Read the model definition and answer for the solid it produces. Units are mm, in the model's axes. A direction names the side the tool comes from. Give positions to 0.01 mm unless a question says otherwise; leave off trailing zeros. Order: outer loops, then holes, each group sorted by start corner. A loop starts at its lowest first (then second) coordinate and runs counter-clockwise, first axis right, second up.
Item 1: The mould has two halves that part along Y. Classify faces 3 (the face through (-35, -635, 1)), 4 (the face through (-26, 381, 12.7)), 5 (the face through (-28, -9, 6.35)), 6 (the face through (-35, 635, 1)): +Y half, -Y half, draft (parallel to the pull), parting line (faces both ways), or undercut.
Item 2: Given pin 1 Ø12.5 at (y, z) = (125, -14) entering from +X; pin 2 Ø1.5 at (x, y) = (-39.5, 37.5) entering from -Z; pin 3 Ø5 at (x, y) = (-39.5, 440.5) entering from +Z, each flat-ended and moving along its own axis, determine where each tip first touches the part or whether it passes through.
Item 3: A cutting plane is placed at B-B (z = -9). Write down the section's boundary in (x, y), plus the area to 3 significant figures.
Item 4: A cutting plane is placed at A-A (y = -316.5). Write down the section's boundary in (x, z), plus the area to 3 significant figures.
Item 5: Which of the six approach directions +Z, -Z, +X, -X, +Y, -Y give full straight-line access (tool end or side, diameter ignored) to faces 1 (the face through (-50.8, -9, -13)), 2 (the face through (-26, -381, 12.7))?
Item 6: Find the intervals of material crossed by line 1 along X through (y, z) = (466.5, -13); line 2 along Z through (x, y) = (-6, 179.5); line 3 along Y through (x, z) = (-35, 11), in increasing order.
from build123d import *

# Parameters (mm, degrees)
F1_DEPTH = 635
F2_R     = 12.7
F3_DEPTH = 12.7


# Not quite as in the source:
# - a fillet or chamfer that OpenCascade refuses, or shapes differently, is made with other operations: its cross-section is extruded or revolved along the edge and cut away or added


with BuildPart() as f1:
    # F0 (on Front) → F1 (new body, symmetric)
    with BuildSketch(Plane.XZ):
        Polygon((-50.8, 0), (0, 0), (0, 6.35), (-57.15, 6.35), (-57.15, -25.4), (-50.8, -25.4), align=None)
    extrude(amount=F1_DEPTH, both=True)

    # F2 (on Top) → F3 (join)
    with BuildSketch(Plane.XY):
        with Locations((-25.4, 381)):
            Circle(F2_R)
        with Locations((-25.4, -381)):
            Circle(F2_R)
    extrude(amount=F3_DEPTH)

    # F4: fillet of radius 7.62 on 1 edges, made by hand

    # F4_s1 → F4_t2 (revolve)
    with BuildSketch(Plane.XZ.offset(-381)):
        with BuildLine():
            ThreePointArc((-5.1865786755, 6.35), (-10.1052675251, 8.1501288674), (-12.7, 12.7))
            Line((-12.7, 12.7), (-12.7, 6.35))
            Line((-12.7, 6.35), (-5.1865786755, 6.35))
        make_face()
    revolve(axis=Axis((-25.4, 381, 6.35), (0, 0, -1)))

    # F5: fillet of radius 7.62 on 1 edges, made by hand

    # F5_s1 → F5_t2 (revolve)
    with BuildSketch(Plane.XZ.offset(381)):
        with BuildLine():
            ThreePointArc((-5.1865786755, 6.35), (-10.1052675251, 8.1501288674), (-12.7, 12.7))
            Line((-12.7, 12.7), (-12.7, 6.35))
            Line((-12.7, 6.35), (-5.1865786755, 6.35))
        make_face()
    revolve(axis=Axis((-25.4, -381, 6.35), (0, 0, -1)))


solid = f1.part
Response values:
1. face 3: -Y half
1. face 4: draft
1. face 5: undercut
1. face 6: +Y half
2. pin 1: stops at x = -50.8
2. pin 2: stops at z = 0
2. pin 3: stops at z = 6.35
3. outline: (-57.15, -635) - (-50.8, -635) - (-50.8, 635) - (-57.15, 635) - close
3. area: 8,060 mm2
4. outline: (-57.15, -25.4) - (-50.8, -25.4) - (-50.8, 0) - (0, 0) - (0, 6.35) - (-57.15, 6.35) - close
4. area: 524 mm2
5. face 1: -Z, +X, +Y, -Y
5. face 2: +Z, +X, -X, +Y, -Y
6. line 1: x = -57.15 to -50.8
6. line 2: z = 0 to 6.35
6. line 3: y = -390.05 to -371.95, 371.95 to 390.05
